The listing builds one solid part. Answer for the finished solid, in the listing's coordinates (mm). Face numbers are marked on the shaded views. Round coordinates to 2 decimals unless told otherwise and drop trailing zeros. Loops run counter-clockwise (first coordinate to the right, second up) from the corner with the lowest first, then second, coordinate; pieces in that order, holes last. Notation, with made-up numbers: (68.25, 63) -> (111.25, 63) arc R9 cw to (111.25, 76) -> close; hole circle Ø10 at (51.5, 55). An arc over 180 degrees is marked (long way). Write each question's results on one line, items separated by ' | '. Start each with the question number.
(1) The part is cut by section A-A (x = 0). Determine the outline of the cut face in (y, z), plus the area to 4 significant figures.
(2) Flat-ended cylindrical pins translate along their axes: pin 1 (2 mm diameter, centred on x = -10.5, z = 1.5, fed in from +Y); pin 2 (1.5 mm diameter, centred on y = 13.5, z = 1.5, fed in from +X). Find the tip coordinate at first contact, or state that the pin passes through.
(3) The part is cut by section C-C (z = 1.6). Determine the outline of the cut face in (x, y), plus the area to 3 significant figures.
(4) Determine the mould class of the marked faces 1, 2 and 3 for opening direction X: released by +X, released by -X, zero draft, split by the parting line, or undercut.
(5) Straight lines are drawn through the part: probe 1 along Y at (x, z) = (0, 2); probe 2 along X at (y, z) = (1.5, 0.4); probe 3 along X at (y, z) = (1.5, 2.1). For each, find the intervals that lie inside material, in ascending order.
```python
from build123d import *

# Parameters (mm, degrees)
SKETCH_1_W              = 25
SKETCH_1_H              = 4
HOLE_WIZARD_5_5_5_5_1_D = 5.5
HOLE_WIZARD_4_5_4_5_1_D = 4.5
CHAMFER_1_SIZE          = 0.5


with BuildPart() as part:
    # 草图1 → 旋转1 (revolve)
    with BuildSketch(Plane(origin=(0, 0, 0), x_dir=(1, 0, 0), z_dir=(0, 1, 0))):
        with Locations((12.5, -2)):
            Rectangle(SKETCH_1_W, SKETCH_1_H)
    revolve(axis=Axis((0, 0, 0), (0, 0, 1)))

    # Ø5.5 (5.5) 直径孔1 (through all)
    with Locations(Plane(origin=(0, 0, 0), x_dir=(-1, 0, 0), z_dir=(0, 0, -1))):
        with Locations((0, 0)):
            Hole(HOLE_WIZARD_5_5_5_5_1_D / 2)

    # Ø4.5 (4.5) 直径孔1 (through all)
    with Locations(Plane(origin=(0, 0, 0), x_dir=(-1, 0, 0), z_dir=(0, 0, -1))):
        with Locations((0, 20), (-20, 0), (0, -20), (20, 0)):
            Hole(HOLE_WIZARD_4_5_4_5_1_D / 2)

    # 倒角1
    chamfer_1_edges = [part.edges().sort_by_distance(p)[0] for p in [
        (-25, 0, 4),
        (-25, 0, 0),
    ]]
    chamfer(chamfer_1_edges, length=CHAMFER_1_SIZE)


solid = part.part
```
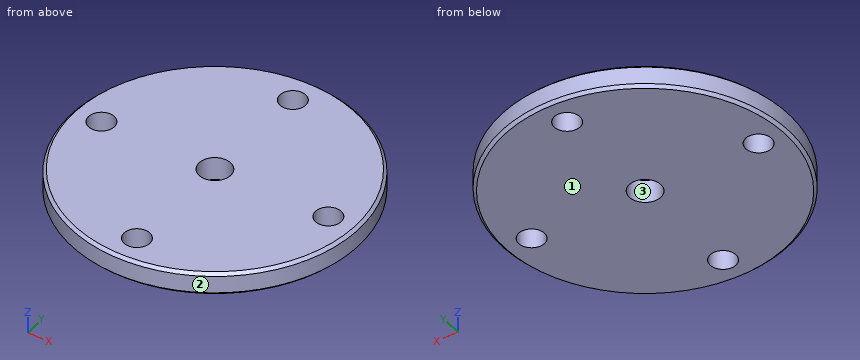
Checked values:
1) outline: (-25, 0.5) -> (-24.5, 0) -> (-22.25, 0) -> (-22.25, 4) -> (-24.5, 4) -> (-25, 3.5) -> close; (-17.75, 0) -> (-2.75, 0) -> (-2.75, 4) -> (-17.75, 4) -> close; (2.75, 0) -> (17.75, 0) -> (17.75, 4) -> (2.75, 4) -> close; (22.25, 0) -> (24.5, 0) -> (25, 0.5) -> (25, 3.5) -> (24.5, 4) -> (22.25, 4) -> close | area: 141.5 mm2
2) pin 1: stops at y = 23.12 | pin 2: stops at x = 21.5
3) outline: circle Ø50 at (0, 0); hole circle Ø4.5 at (-20, 0); hole circle Ø5.5 at (0, 0); hole circle Ø4.5 at (0, -20); hole circle Ø4.5 at (0, 20); hole circle Ø4.5 at (20, 0) | area: 1,880 mm2
4) face 1: zero draft | face 2: split by the parting line | face 3: undercut
5) probe 1: y = -25 to -22.25, -17.75 to -2.75, 2.75 to 17.75, 22.25 to 25 | probe 2: x = -24.85 to -21.68, -18.32 to -2.3, 2.3 to 18.32, 21.68 to 24.85 | probe 3: x = -24.95 to -21.68, -18.32 to -2.3, 2.3 to 18.32, 21.68 to 24.95
